from build123d import *

# Parameters (mm, degrees)
EXTRUDE1_DEPTH               = 1.5875
CHAMFER1_SIZE                = 1.397
F_10_0_1935_DIAMETER_HOLE1_D = 4.9149
LPATTERN2_COUNT              = 3
LPATTERN2_PITCH              = 101.6
LPATTERN2_COL_COUNT          = 2
LPATTERN2_COL_PITCH          = 101.6


with BuildPart() as part:
    # Sketch1 → Extrude1 (new, symmetric)
    with BuildSketch(Plane.XY):
        Polygon((0, 0), (193.675, 0), (101.6, 152.4), (0, 152.4), (-101.6, 152.4), (-193.675, 0), align=None)
    extrude(amount=EXTRUDE1_DEPTH, both=True)

    # Chamfer1
    chamfer1_edges = [part.edges().sort_by_distance(p)[0] for p in [
        (147.6375, 76.2, 1.5875),
        (-147.6375, 76.2, 1.5875),
        (-147.6375, 76.2, -1.5875),
        (147.6375, 76.2, -1.5875),
    ]]
    chamfer(chamfer1_edges, length=CHAMFER1_SIZE)

    # #10 (0.1935) Diameter Hole1 (through all)
    with Locations(Plane(origin=(50.8, 8.5852, 1.5875), x_dir=(1, 0, 0), z_dir=(0, 0, 1))):
        with Locations((0, 0)):
            f_10_0_1935_diameter_hole1 = Hole(F_10_0_1935_DIAMETER_HOLE1_D / 2)

    # LPattern2: #10 (0.1935) Diameter Hole1 ×3
    with Locations(*[(-i * LPATTERN2_PITCH, 0, 0) for i in range(1, LPATTERN2_COUNT)]):
        add(f_10_0_1935_diameter_hole1, mode=Mode.SUBTRACT)

    # LPattern2 col: #10 (0.1935) Diameter Hole1 ×2
    with Locations(*[(i * LPATTERN2_COL_PITCH, 0, 0) for i in range(1, LPATTERN2_COL_COUNT)]):
        add(f_10_0_1935_diameter_hole1, mode=Mode.SUBTRACT)


solid = part.part
Verification items for the finished model (mm, model axes). Give positions to 0.01 mm unless a question says otherwise; leave off trailing zeros. Order: outer loops, then holes, each group sorted by start corner. A loop starts at its lowest first (then second) coordinate and runs counter-clockwise, first axis right, second up. Notation, with made-up numbers: M 83,-8.75 L 138,-8.75 A31 cw 138,28.25 Z; hole C 69.5,-20 d5. An arc over 180 degrees is marked long. Answer as a JSON object with one key per item and string values. Group by question number.
1) Cross-section at C-C (x = -136). Enter the section's corners in (y, z).
2) Depth check by flat-ended pin: pin 1 Ø1.5 at (y, z) = (94, 0.5) entering from -X. Enter the tip coordinate at first touch or a pass-through.
3) Cross-section at D-D (y = 28). Enter the section's corners in (x, z), then the cut area to 3 significant figures.
4) Cross-section at B-B (y = 61). Enter the section's corners in (x, z).
5) Scan lines: line 1 along Y through (x, z) = (50.8, -0.2); line 2 along X through (y, z) = (9, -1.15); line 3 along X through (y, z) = (8, -0.2). Record each from-to range of solid material in increasing order. Write a range as [from, to].
6) Cross-section at A-A (z = -0.8). Enter the section's corners in (x, y), then the cut area to 3 significant figures.
Result sheet:
{
 "1": {"outline": "M 0,-1.59 L 92.76,-1.59 L 95.46,-0.19 L 95.46,0.19 L 92.76,1.59 L 0,1.59 Z"},
 "2": {"pin 1": "stops at x = -137.3"},
 "3": {"outline": "M -176.76,-0.19 L -175.13,-1.59 L 175.13,-1.59 L 176.76,-0.19 L 176.76,0.19 L 175.13,1.59 L -175.13,1.59 L -176.76,0.19 Z", "area": "1,120 mm2"},
 "4": {"outline": "M -156.82,-0.19 L -155.19,-1.59 L 155.19,-1.59 L 156.82,-0.19 L 156.82,0.19 L 155.19,1.59 L -155.19,1.59 L -156.82,0.19 Z"},
 "5": {"line 1": "y = [0, 6.13], [11.04, 152.4]", "line 2": "x = [-187.12, -154.82], [-149.98, -53.22], [-48.38, 48.38], [53.22, 149.98], [154.82, 187.12]", "line 3": "x = [-188.83, -154.79], [-150.01, -53.19], [-48.41, 48.41], [53.19, 150.01], [154.79, 188.83]"},
 "6": {"outline": "M -192.96,0 L 192.96,0 L 100.89,152.4 L -100.89,152.4 Z; hole C -152.4,8.59 d4.91; hole C -50.8,8.59 d4.91; hole C 50.8,8.59 d4.91; hole C 152.4,8.59 d4.91", "area": "44,700 mm2"}
}
